Could you check a few things on this model? Use its own coordinates, in mm. Face numbers are marked on the shaded views. A direction names the side the tool comes from. Round coordinates to 2 decimals unless told otherwise and drop trailing zeros. Write each loop counter-clockwise with the first axis right and the second up, starting at its lowest first coordinate (ties: lowest second). Pieces come first, ordered by that corner, then holes. Notation, with made-up numbers: M 25,76 L 48,76 A16 ccw 48,83 Z; hole C 65,-25 d4. An arc over 180 degrees is marked long. One line per item, written item: value. Start each with the question number.
(1) If I drill on L1, parallel to Y at x = 14.5, z = -36.78; L2, parallel to Z at x = 13.25, y = 0; L3, parallel to Z at x = -15, y = -5.25, over which ranges is the centre line in solid material (lowest first)?
(2) I want a section at B-B on z = 53.5. Please give me the cut outline in (x, y), and give its area (3 significant figures).
(3) Which directions (+Z, -Z, +X, -X, +Y, -Y) give clear straight access to the entire face, cutting with the end or side of a thin tool? Please do the marked faces 4, 5, 6, 7 and 8.
(4) I'm going to push flat-ended pins straight in: pin 1 Ø4 at (x, z) = (-12.5, 3) entering from -Y; pin 2 Ø4 at (x, y) = (-15.5, 0.5) entering from +Z; pin 3 Ø10 at (y, z) = (-4.5, -3.5) entering from -X; pin 4 Ø3.5 at (y, z) = (1.5, -52.5) entering from +X. Where does each tip first touch, or does it pass through?
(5) Thinking about a two-plate mould opening in Y: for the marked faces 1, 2 and 3, which applies, released by +Y, released by -Y, zero draft, split by the parting line, or undercut?
(6) I want a section at A-A on x = 13. Please give me the cut outline in (y, z), and give its area (3 significant figures).
(7) I want a section at C-C on y = 0. Count the separate pieces of the cut face and the enclosed holes in it, and give its area (3 significant figures).
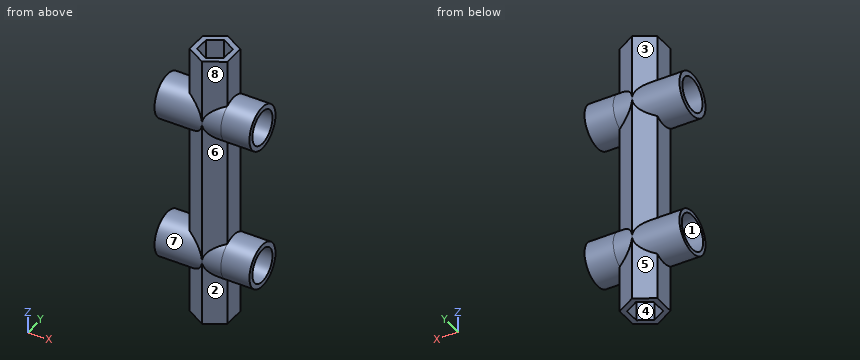
```python
from build123d import *

# Parameters (mm, degrees)
BOSS_EXTRUDE2_DEPTH      = 70
CUT_EXTRUDE6_DEPTH       = 15
CUT_EXTRUDE7_DEPTH       = 15
SKETCH3_R                = 11
SKETCH3_R_2              = 8.5
BOSS_EXTRUDE3_DEPTH      = 14.5
BOSS_EXTRUDE3_DEPTH_BACK = 33.5
SKETCH12_R               = 8.5
SKETCH12_R_2             = 9
CUT_EXTRUDE8_DEPTH       = 34.5


with BuildPart() as part:
    # Sketch1_3 → Boss-Extrude2 (new body, symmetric)
    with BuildSketch(Plane.XY):
        Polygon((0, -11), (9.526279442, -5.5), (9.526279442, 5.5), (0, 11), (-9.526279442, 5.5), (-9.526279442, -5.5), align=None)
    extrude(amount=BOSS_EXTRUDE2_DEPTH, both=True)

    # Sketch10 → Cut-Extrude6 (cut)
    with BuildSketch(Plane.XY.offset(70)):
        Polygon((0.040785795, -7.840785795), (6.795783944, -3.940785795), (6.795783944, 3.859214205), (0.040785795, 7.759214205), (-6.714212355, 3.859214205), (-6.714212355, -3.940785795), align=None)
    extrude(amount=-CUT_EXTRUDE6_DEPTH, mode=Mode.SUBTRACT)

    # Sketch11 → Cut-Extrude7 (cut)
    with BuildSketch(Plane(origin=(0, 0, -70), x_dir=(-1, 0, 0), z_dir=(0, 0, -1))):
        Polygon((0, -7.820392897), (6.75499815, -3.920392897), (6.75499815, 3.879607103), (0, 7.779607103), (-6.75499815, 3.879607103), (-6.75499815, -3.920392897), align=None)
    extrude(amount=-CUT_EXTRUDE7_DEPTH, mode=Mode.SUBTRACT)

    # Sketch3 → Boss-Extrude3 (add, two sides)
    with BuildSketch(Plane(origin=(9.526279442, 0, 0), x_dir=(0, 0, -1), z_dir=(1, 0, 0))) as boss_extrude3_sk:
        with Locations((-36.78, 0)):
            Circle(SKETCH3_R)
        with Locations((-36.78, 0)):
            Circle(SKETCH3_R_2, mode=Mode.SUBTRACT)
        with Locations((36.78, 0)):
            Circle(SKETCH3_R)
        with Locations((36.78, 0)):
            Circle(SKETCH3_R_2, mode=Mode.SUBTRACT)
    extrude(amount=BOSS_EXTRUDE3_DEPTH)
    extrude(boss_extrude3_sk.sketch, amount=-BOSS_EXTRUDE3_DEPTH_BACK)

    # Sketch12 → Cut-Extrude8 (cut, through all)
    with BuildSketch(Plane(origin=(9.526279442, 0, 0), x_dir=(0, 0, -1), z_dir=(1, 0, 0))):
        with Locations((-36.78, 0)):
            Circle(SKETCH12_R)
        with Locations((36.78, 0)):
            Circle(SKETCH12_R_2)
    extrude(amount=-CUT_EXTRUDE8_DEPTH, mode=Mode.SUBTRACT)


solid = part.part
```
Found:
1. L1: y = -11 to -8.5, 8.5 to 11
1. L2: z = -47.78 to -45.28, -28.28 to -25.78, 25.78 to 28.28, 45.28 to 47.78
1. L3: z = -46.45 to -44.09, -29.47 to -27.11, 27.11 to 30.1, 43.46 to 46.45
2. outline: M -9.53,-5.5 L 0,-11 L 9.53,-5.5 L 9.53,5.5 L 0,11 L -9.53,5.5 Z
2. area: 314 mm²
3. face 4: -Z
3. face 5: -Z, -X, +Y
3. face 6: +X, -Y
3. face 7: -X
3. face 8: +Z, +X, -Y
4. pin 1: passes through
4. pin 2: stops at z = 47.78
4. pin 3: stops at x = -9.53
4. pin 4: stops at x = 9.53
5. face 1: undercut
5. face 2: released by -Y
5. face 3: released by +Y
6. outline: C 0,-36.78 d22; C 0,36.78 d22; hole C 0,-36.78 d17; hole C 0,36.78 d17
6. area: 306 mm²
7. separate pieces: 3
7. enclosed holes: 0
7. area: 1,870 mm²
